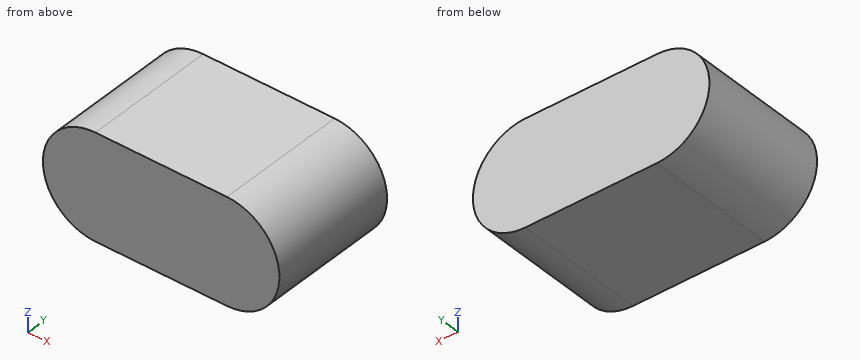
```python
from build123d import *

# Parameters (mm, degrees)
CYLINDER103_R     = 4
CYLINDER103_DEPTH = 10
CYLINDER104_R     = 4
CYLINDER104_DEPTH = 10
BOX069_W          = 10
BOX069_H          = 10
BOX069_DEPTH      = 8


with BuildPart() as obj1:
    # Cylinder103 → Cylinder103 (new body)
    with BuildSketch(Plane(origin=(65, 10, 23.5), x_dir=(1, 0, 0), z_dir=(0, -1, 0))):
        Circle(CYLINDER103_R)
    extrude(amount=CYLINDER103_DEPTH)


with BuildPart() as obj2:
    # Cylinder104 → Cylinder104 (new body)
    with BuildSketch(Plane(origin=(75, 10, 23.5), x_dir=(1, 0, 0), z_dir=(0, -1, 0))):
        Circle(CYLINDER104_R)
    extrude(amount=CYLINDER104_DEPTH)


with BuildPart() as obj3:
    # Box069 → Box069 (new body)
    with BuildSketch(Plane(origin=(65, 0, 19.5), x_dir=(1, 0, 0), z_dir=(0, 0, 1))):
        with Locations((5, 5)):
            Rectangle(BOX069_W, BOX069_H)
    extrude(amount=BOX069_DEPTH)

    # Fusion047: union obj1, obj2
    add(obj1.part)
    add(obj2.part)


solid = obj3.part
```
Geometry: final body of the model. Coordinates: model frame, mm. Coordinates: 2 decimals unless noted, no trailing zeros. Loops run counter-clockwise (first coordinate to the right, second up) from the corner with the lowest first, then second, coordinate; pieces in that order, holes last. Notation, with made-up numbers: (34, 34) -> (39, 34) arc R6 ccw to (39, 41) -> close; hole circle Ø7 at (83, 25). An arc over 180 degrees is marked (long way). Use a Markdown table: item, result. Add a question column.
(1) Line query: line 1 along Z through (x, y) = (63, 4.5); line 2 along X through (y, z) = (6, 20.5); line 3 along X through (y, z) = (4, 26.25). Output: solid intervals per line, ascending.
(2) Pin query (flat end, axial travel): pin 1 Ø1 at (x, y) = (76, 2.5) entering from -Z; pin 2 Ø2 at (x, z) = (67.5, 20.5) entering from -Y. Return the tip coordinate at first contact, or that it passes through.
(3) Section query B-B, the plane z = 25. Return loops of the section in (x, y), plus the area to 3 significant figures.
(4) Section query A-A, the plane y = 1.5. Return loops of the section in (x, z), plus the area to 3 significant figures.
Answer:
| question | item | result |
|---|---|---|
| 1 | line 1 | z = 20.04 to 26.96 |
| 1 | line 2 | x = 62.35 to 77.65 |
| 1 | line 3 | x = 62.1 to 77.9 |
| 2 | pin 1 | stops at z = 19.53 |
| 2 | pin 2 | stops at y = 0 |
| 3 | outline | (61.29, 0) -> (78.71, 0) -> (78.71, 10) -> (61.29, 10) -> close |
| 3 | area | 174 mm^2 |
| 4 | outline | (65, 19.5) -> (75, 19.5) arc R4 ccw to (75, 27.5) -> (65, 27.5) arc R4 ccw to start |
| 4 | area | 130 mm^2 |
